CAD build for the part. Positions are in the model's coordinates, mm. Face numbers are marked on the shaded views. A direction names the side the tool comes from. Coordinates: 2 decimals unless noted, no trailing zeros. Write each loop counter-clockwise with the first axis right and the second up, starting at its lowest first coordinate (ties: lowest second). Pieces come first, ordered by that corner, then holes. Notation, with made-up numbers: (1.5, 21) - (22.5, 21) arc R25 ccw to (22.5, 36) - close; hole circle Ø9 at (12, 25). An arc over 180 degrees is marked (long way). One line per question, with ' | ' between items. Start each with the question number.
1. Flat gauge pins, fed straight in: P1, Ø3, axis at x = -7, y = 7, coming from the +Z side; P2, Ø2, axis at x = 5, y = 5.5, coming from the -Z side; P3, Ø8, axis at x = 0, z = 0, coming from the -Y side; P4, Ø2, axis at y = 3.5, z = 6.5, coming from the +X side. Where does each tip first touch, or does it go through?
2. Which spindle directions (+Z, -Z, +X, -X, +Y, -Y) get a long thin tool onto all of the face, cutting with end or side? Do the marked faces 4, 5 and 6. Say none if no direction does.
3. Two-plate mould, pull along Z, no slides. Class the marked faces 1, 2 and 3: +Z half, -Z half, draft (parallel to the pull), parting line (faces both ways), or undercut.
4. Probe line 1 (X direction, y = 0.4, z = 0); line 2 (X direction, y = 4.5, z = 0); line 3 (Y direction, x = -1.75, z = -10). List the from-to ranges inside material, lowest first.
5. Band-saw the part on A-A, the plane y = 7. Write the cut outline in (x, z).
from build123d import *

# Parameters (mm, degrees)
SKETCH1_R           = 13
SKETCH1_R_2         = 5
BOSS_EXTRUDE1_DEPTH = 8
SKETCH2_R           = 11
SKETCH2_R_2         = 6
CUT_EXTRUDE1_DEPTH  = 0.5
CUT_EXTRUDE2_START  = -7.5
SKETCH2_2_R         = 11
SKETCH2_2_R_2       = 6
CUT_EXTRUDE2_DEPTH  = 0.5
CHAMFER1_SIZE       = 0.2


with BuildPart() as part:
    # Sketch1 → Boss-Extrude1 (new body)
    with BuildSketch(Plane(origin=(0, 0, 0), x_dir=(1, 0, 0), z_dir=(0, 1, 0))):
        with Locations(Location((0, 0, 0), (0, 0, 270))):
            Circle(SKETCH1_R)
        with Locations(Location((0, 0, 0), (0, 0, 270))):
            Circle(SKETCH1_R_2, mode=Mode.SUBTRACT)
    extrude(amount=BOSS_EXTRUDE1_DEPTH)

    # Sketch2 → Cut-Extrude1 (cut)
    with BuildSketch(Plane(origin=(0, 8, 0), x_dir=(1, 0, 0), z_dir=(0, 1, 0))):
        with Locations(Location((0, 0, 0), (0, 0, 270))):
            Circle(SKETCH2_R)
        with Locations(Location((0, 0, 0), (0, 0, 270))):
            Circle(SKETCH2_R_2, mode=Mode.SUBTRACT)
    extrude(amount=-CUT_EXTRUDE1_DEPTH, mode=Mode.SUBTRACT)

    # Sketch2<2> → Cut-Extrude2 (cut)
    with BuildSketch(Plane(origin=(0, 8, 0), x_dir=(1, 0, 0), z_dir=(0, 1, 0)).offset(CUT_EXTRUDE2_START)):
        with Locations(Location((0, 0, 0), (0, 0, 270))):
            Circle(SKETCH2_2_R)
        with Locations(Location((0, 0, 0), (0, 0, 270))):
            Circle(SKETCH2_2_R_2, mode=Mode.SUBTRACT)
    extrude(amount=-CUT_EXTRUDE2_DEPTH, mode=Mode.SUBTRACT)

    # Chamfer1
    chamfer1_edges = [part.edges().sort_by_distance(p)[0] for p in [
        (0, 8, -11),
        (0, 8, -6),
        (0, 0, -6),
        (0, 0, -11),
        (0, 0, -13),
        (0, 8, -13),
    ]]
    chamfer(chamfer1_edges, length=CHAMFER1_SIZE)


solid = part.part
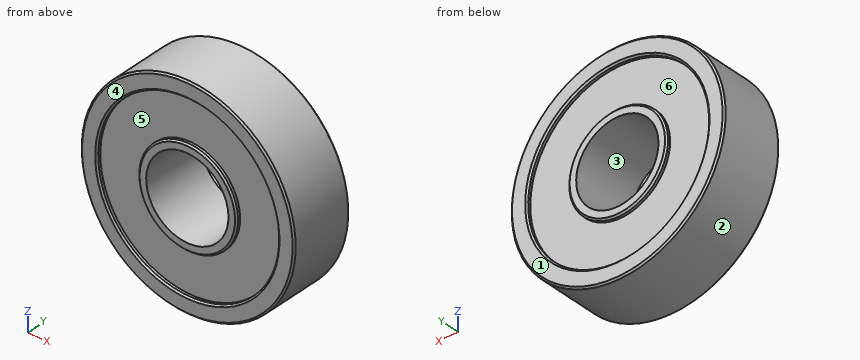
Filled in:
1) P1: stops at z = 11.78 | P2: stops at z = -12.37 | P3: passes through | P4: stops at x = 11.78
2) face 4: +Z, -Z, +X, -X, -Y | face 5: -Y | face 6: +Y
3) face 1: draft | face 2: parting line | face 3: undercut
4) line 1: x = -13 to -11, -6 to -5, 5 to 6, 11 to 13 | line 2: x = -13 to -5, 5 to 13 | line 3: y = 0.5 to 7.5
5) outline: circle Ø26 at (0, 0); hole circle Ø10 at (0, 0)
